Can you work these out from the model? Positions are in its coordinate system, mm. A direction names the side the tool comes from. Give positions to 0.01 mm unless a question says otherwise; leave off trailing zeros. Order: outer loops, then holes, each group sorted by start corner. A loop starts at its lowest first (then second) coordinate and runs counter-clockwise, first axis right, second up.
Item 1: I'm going to push flat-ended pins straight in: pin 1 Ø1.2 at (x, z) = (-32.5, 8.5) entering from +Y; pin 2 Ø8 at (y, z) = (-13, 0.5) entering from -X; pin 3 Ø5.5 at (y, z) = (30.5, 8.5) entering from -X. Where does each tip first touch, or does it pass through?
Item 2: Which directions (+Z, -Z, +X, -X, +Y, -Y) give clear straight access to the entire face, cutting with the end or side of a thin tool? Please do faces 4 (the flat face through (-21, -55, 14.5)), 5 (the flat face through (-21, -73, 16)), 6 (the flat face through (-33, -36.914, 10)), 7 (the flat face through (-21, 7, 4)).
Item 3: I want a section at A-A, the plane y = 16.5. Write out the boundary of the cut face in (x, z), then the cut area to 3 significant figures.
Item 4: If we mould it in two halves opening along X, with no side actions, what happens to faces 1 (the flat face through (0, 48.37, 11)), 2 (the flat face through (22.5, -15, 16)), 3 (the cylindrical face through (-16.291, -75.643, 9.93))? For each: +X half, -X half, draft (parallel to the pull), parting line (faces both ways), or undercut.
Item 5: If I drill on line 1 along X through (y, z) = (-12, -2.75); line 2 along X through (y, z) = (0, 12.25); line 3 along Y through (x, z) = (14.5, 1.95), over which ranges is the centre line in solid material (lowest first)?
```python
from build123d import *

# Parameters (mm, degrees)
CROQUIS1_W               = 38
CROQUIS1_H               = 81
CROQUIS1_W_2             = 27
CROQUIS1_H_2             = 72
CROQUIS1_H_3             = 38
CROQUIS1_R               = 3.5
SALIENTE_EXTRUIR1_DEPTH  = 5
CROQUIS2_W               = 38
CROQUIS2_H               = 81
CROQUIS2_W_2             = 27
CROQUIS2_H_2             = 72
SALIENTE_EXTRUIR2_DEPTH  = 5
SALIENTE_EXTRUIR9_START  = -1
SALIENTE_EXTRUIR9_DEPTH  = 1
SALIENTE_EXTRUIR10_DEPTH = 11
SALIENTE_EXTRUIR11_DEPTH = 10
REDONDEO1_R              = 1
REDONDEO2_R              = 1
REDONDEO3_R              = 1
CROQUIS6_W               = 6
CROQUIS6_H               = 9
CORTAR_EXTRUIR1_DEPTH    = 8
CROQUIS7_W               = 6
CROQUIS7_H               = 9
CROQUIS7_R               = 2.5
SALIENTE_EXTRUIR12_DEPTH = 3
SALIENTE_EXTRUIR13_DEPTH = 11
REDONDEO4_R              = 5
CROQUIS9_R               = 0.6
CORTAR_EXTRUIR2_DEPTH    = 80
SALIENTE_EXTRUIR14_START = -2.5
CROQUIS10_R              = 0.6
SALIENTE_EXTRUIR14_DEPTH = 2.5
CROQUIS11_R              = 4
CROQUIS11_R_2            = 3.5
CROQUIS11_R_3            = 2.5
CROQUIS11_R_4            = 2
CORTAR_EXTRUIR3_DEPTH    = 1
SALIENTE_EXTRUIR15_DEPTH = 3
CROQUIS14_R              = 1.5
CORTAR_EXTRUIR4_DEPTH    = 14
CROQUIS16_W              = 3.5
CROQUIS16_H              = 3
SALIENTE_EXTRUIR16_DEPTH = 4
CROQUIS25_R              = 3
CROQUIS25_R_2            = 1.5
SALIENTE_EXTRUIR21_DEPTH = 18
CROQUIS26_R              = 1.5
CORTAR_EXTRUIR7_DEPTH    = 18
CROQUIS28_R              = 1
CORTAR_EXTRUIR8_DEPTH    = 4


with BuildPart() as part:
    # Croquis1 → Saliente-Extruir1 (new body)
    # profile 1 of 5: a face of its own
    with BuildSketch(Plane.XY):
        Rectangle(CROQUIS1_W, CROQUIS1_H)
        Rectangle(CROQUIS1_W_2, CROQUIS1_H_2, mode=Mode.SUBTRACT)
    # profile 2 of 5: a face of its own
    with BuildSketch(Plane.XY):
        with Locations((0, -59.5)):
            Rectangle(CROQUIS1_W, CROQUIS1_H_3)
        with Locations((-9.5, -69)):
            Circle(CROQUIS1_R, mode=Mode.SUBTRACT)
        with Locations((9.5, -59.5)):
            Circle(CROQUIS1_R, mode=Mode.SUBTRACT)
        with Locations((-9.5, -50)):
            Circle(CROQUIS1_R, mode=Mode.SUBTRACT)
    # profile 3 of 5: a face of its own
    with BuildSketch(Plane.XY):
        with BuildLine():
            ThreePointArc((19, -78.5), (26.870057685, -59.5), (19, -40.5))
            Line((19, -40.5), (19, -78.5))
        make_face()
    # profile 4 of 5: a face of its own
    with BuildSketch(Plane.XY):
        with BuildLine():
            Line((19, -78.5), (-19, -78.5))
            ThreePointArc((-19, -78.5), (0, -86.370057685), (19, -78.5))
        make_face()
    # profile 5 of 5: a face of its own
    with BuildSketch(Plane.XY):
        with BuildLine():
            Line((-19, -78.5), (-19, -40.5))
            ThreePointArc((-19, -40.5), (-26.870057685, -59.5), (-19, -78.5))
        make_face()
    extrude(amount=SALIENTE_EXTRUIR1_DEPTH)

    # Croquis2 → Saliente-Extruir2 (add)
    with BuildSketch(Plane(origin=(0, 0, 0), x_dir=(-1, 0, 0), z_dir=(0, 0, -1))):
        Rectangle(CROQUIS2_W, CROQUIS2_H)
        Rectangle(CROQUIS2_W_2, CROQUIS2_H_2, mode=Mode.SUBTRACT)
    extrude(amount=SALIENTE_EXTRUIR2_DEPTH)

    # Croquis3 → Saliente-Extruir9 (add)
    with BuildSketch(Plane.XY.offset(5).offset(SALIENTE_EXTRUIR9_START)):
        with BuildLine():
            Line((26.870057685, -59.5), (26.870057685, 40.5))
            Line((26.870057685, 40.5), (19, 48.370057685))
            Line((19, 48.370057685), (-19, 48.370057685))
            Line((-19, 48.370057685), (-26.870057685, 40.5))
            Line((-26.870057685, 40.5), (-26.870057685, -59.5))
            ThreePointArc((-26.870057685, -59.5), (0, -86.370057685), (26.870057685, -59.5))
        make_face()
        with BuildLine():
            Line((19, -59.5), (19, 40.5))
            Line((19, 40.5), (-19, 40.5))
            Line((-19, 40.5), (-19, -59.5))
            ThreePointArc((-19, -59.5), (0, -78.5), (19, -59.5))
        make_face(mode=Mode.SUBTRACT)
    extrude(amount=SALIENTE_EXTRUIR9_DEPTH)

    # Croquis4 → Saliente-Extruir10 (add)
    with BuildSketch(Plane(origin=(0, 0, 4), x_dir=(-1, 0, 0), z_dir=(0, 0, -1))):
        with BuildLine():
            Line((19, 40.5), (19, -40.5))
            ThreePointArc((19, -40.5), (24.824696333, -49.217274097), (26.870057685, -59.5))
            Line((26.870057685, -59.5), (26.870057685, 40.5))
            Line((26.870057685, 40.5), (19, 48.370057685))
            Line((19, 48.370057685), (-19, 48.370057685))
            Line((-19, 48.370057685), (-26.870057685, 40.5))
            Line((-26.870057685, 40.5), (-26.870057685, -59.5))
            ThreePointArc((-26.870057685, -59.5), (-24.824696333, -49.217274097), (-19, -40.5))
            Line((-19, -40.5), (-19, 40.5))
            Line((-19, 40.5), (19, 40.5))
        make_face()
    extrude(amount=-SALIENTE_EXTRUIR10_DEPTH)

    # Croquis5 → Saliente-Extruir11 (add)
    with BuildSketch(Plane.XY.offset(5)):
        with BuildLine():
            Line((-19, -59.5), (-19, -69))
            ThreePointArc((-19, -69), (-16.217514421, -75.717514421), (-9.5, -78.5))
            Line((-9.5, -78.5), (9.5, -78.5))
            ThreePointArc((9.5, -78.5), (16.217514421, -75.717514421), (19, -69))
            Line((19, -69), (19, -59.5))
            Line((19, -59.5), (19, -40.5))
            ThreePointArc((19, -40.5), (0, -86.370057685), (-19, -40.5))
            Line((-19, -40.5), (-19, -59.5))
        make_face()
    extrude(amount=SALIENTE_EXTRUIR11_DEPTH)

    # Redondeo1
    redondeo1_edges = [part.edges().sort_by_distance(p)[0] for p in [
        (19, -40.5, -2.5),
        (-19, -40.5, -2.5),
        (19, 40.5, -0.5),
        (-19, 40.5, -0.5),
    ]]
    fillet(redondeo1_edges, radius=REDONDEO1_R)

    # Redondeo2
    redondeo2_edges = [part.edges().sort_by_distance(p)[0] for p in [
        (-19, -0.5, 4),
        (0, 40.5, 4),
        (-18.707106781, 40.207106781, 4),
        (18.707106781, 40.207106781, 4),
        (19, -0.5, 4),
    ]]
    fillet(redondeo2_edges, radius=REDONDEO2_R)

    # Redondeo3
    redondeo3_edges = [part.edges().sort_by_distance(p)[0] for p in [
        (19, 48.370057685, 9.5),
        (26.870057685, 40.5, 9.5),
        (-26.870057685, 40.5, 9.5),
        (-19, 48.370057685, 9.5),
    ]]
    fillet(redondeo3_edges, radius=REDONDEO3_R)

    # Croquis6 → Cortar-Extruir1 (cut)
    with BuildSketch(Plane.ZY.offset(26.870057685)):
        with Locations((11.5, -55)):
            Rectangle(CROQUIS6_W, CROQUIS6_H)
    extrude(amount=-CORTAR_EXTRUIR1_DEPTH, mode=Mode.SUBTRACT)

    # Croquis7 → Saliente-Extruir12 (add)
    with BuildSketch(Plane.ZY.offset(26.870057685)):
        with Locations((11.5, -55)):
            Rectangle(CROQUIS7_W, CROQUIS7_H)
        with Locations((11.5, -55)):
            Circle(CROQUIS7_R, mode=Mode.SUBTRACT)
    extrude(amount=-SALIENTE_EXTRUIR12_DEPTH)

    # Croquis8 → Saliente-Extruir13 (add)
    with BuildSketch(Plane.ZY.offset(26.870057685)):
        Polygon((15, 40.085786438), (4, 40.085786438), (4, 37.085786438), (9.5, 37.085786438), (15, 37.085786438), align=None)
        Polygon((9.5, 15.085786438), (4, 15.085786438), (4, 12.085786438), (9.5, 12.085786438), (15, 12.085786438), (15, 15.085786438), align=None)
        Polygon((9.5, -10.914213562), (4, -10.914213562), (4, -13.914213562), (9.5, -13.914213562), (15, -13.914213562), (15, -10.914213562), align=None)
        Polygon((9.5, -36.914213562), (4, -36.914213562), (4, -39.914213562), (15, -39.914213562), (15, -36.914213562), align=None)
    extrude(amount=SALIENTE_EXTRUIR13_DEPTH)

    # Redondeo4
    redondeo4_edges = [part.edges().sort_by_distance(p)[0] for p in [
        (-37.870057685, 38.585786438, 4),
        (-37.870057685, 38.585786438, 15),
        (-37.870057685, 13.585786438, 4),
        (-37.870057685, 13.585786438, 15),
        (-37.870057685, -12.414213562, 4),
        (-37.870057685, -12.414213562, 15),
        (-37.870057685, -38.414213562, 4),
        (-37.870057685, -38.414213562, 15),
    ]]
    fillet(redondeo4_edges, radius=REDONDEO4_R)

    # Croquis9 → Cortar-Extruir2 (cut)
    with BuildSketch(Plane(origin=(0, 40.085786438, 0), x_dir=(1, 0, 0), z_dir=(0, 1, 0))):
        with Locations(Location((-32.370057685, -9.5, 0), (0, 0, 270))):
            Circle(CROQUIS9_R)
    extrude(amount=-CORTAR_EXTRUIR2_DEPTH, mode=Mode.SUBTRACT)

    # Croquis10 → Saliente-Extruir14 (add)
    with BuildSketch(Plane.XZ.offset(39.914213562).offset(SALIENTE_EXTRUIR14_START)):
        with Locations(Location((-32.370057685, 9.5, 0), (0, 0, 90))):
            Circle(CROQUIS10_R)
    extrude(amount=SALIENTE_EXTRUIR14_DEPTH)

    # Croquis11 → Cortar-Extruir3 (cut)
    # profile 1 of 2: a face of its own
    with BuildSketch(Plane(origin=(0, -36.914213562, 0), x_dir=(1, 0, 0), z_dir=(0, 1, 0))):
        with Locations(Location((-32.370057685, -9.5, 0), (0, 0, 270))):
            Circle(CROQUIS11_R)
        with Locations(Location((-32.370057685, -9.5, 0), (0, 0, 270))):
            Circle(CROQUIS11_R_2, mode=Mode.SUBTRACT)
    # profile 2 of 2: a face of its own
    with BuildSketch(Plane(origin=(0, -36.914213562, 0), x_dir=(1, 0, 0), z_dir=(0, 1, 0))):
        with Locations(Location((-32.370057685, -9.5, 0), (0, 0, 270))):
            Circle(CROQUIS11_R_3)
        with Locations(Location((-32.370057685, -9.5, 0), (0, 0, 270))):
            Circle(CROQUIS11_R_4, mode=Mode.SUBTRACT)
    extrude(amount=-CORTAR_EXTRUIR3_DEPTH, mode=Mode.SUBTRACT)

    # Croquis13 → Saliente-Extruir15 (add)
    with BuildSketch(Plane.XY.offset(15)):
        Polygon((-19, -65.5), (-19, 40.5), (-22.5, 40.5), (-22.5, -69), (-19, -69), align=None)
        Polygon((22.5, 40.5), (19, 40.5), (19, -65.5), (19, -69), (22.5, -69), align=None)
        with BuildLine():
            Line((-19, 40.5), (19, 40.5))
            Line((19, 40.5), (22.5, 40.5))
            Line((22.5, 40.5), (22.5, 44.870057685))
            Line((22.5, 44.870057685), (19.292893219, 48.077164466))
            ThreePointArc((19.292893219, 48.077164466), (18.96846987, 48.293937218), (18.585786438, 48.370057685))
            Line((18.585786438, 48.370057685), (-18.585786438, 48.370057685))
            ThreePointArc((-18.585786438, 48.370057685), (-18.96846987, 48.293937218), (-19.292893219, 48.077164466))
            Line((-19.292893219, 48.077164466), (-22.5, 44.870057685))
            Line((-22.5, 44.870057685), (-22.5, 40.5))
            Line((-22.5, 40.5), (-19, 40.5))
        make_face()
    extrude(amount=SALIENTE_EXTRUIR15_DEPTH)

    # Croquis14 → Cortar-Extruir4 (cut)
    with BuildSketch(Plane(origin=(0, 0, 4), x_dir=(-1, 0, 0), z_dir=(0, 0, -1))):
        with Locations((10, 45.370057685)):
            Circle(CROQUIS14_R)
        with Locations(Location((-10, 45.370057685, 0), (0, 0, 180))):
            Circle(CROQUIS14_R)
    extrude(amount=-CORTAR_EXTRUIR4_DEPTH, mode=Mode.SUBTRACT)

    # Croquis16 → Saliente-Extruir16 (add)
    with BuildSketch(Plane(origin=(0, -69, 0), x_dir=(-1, 0, 0), z_dir=(0, -1, 0))):
        with Locations((20.75, -16.5)):
            Rectangle(CROQUIS16_W, CROQUIS16_H)
        with Locations((-20.75, -16.5)):
            Rectangle(CROQUIS16_W, CROQUIS16_H)
    extrude(amount=SALIENTE_EXTRUIR16_DEPTH)

    # Croquis25 → Saliente-Extruir21 (add)
    with BuildSketch(Plane.XY.offset(18)):
        with Locations((0, -70.629942315)):
            Circle(CROQUIS25_R)
        with Locations((0, -70.629942315)):
            Circle(CROQUIS25_R_2, mode=Mode.SUBTRACT)
    extrude(amount=-SALIENTE_EXTRUIR21_DEPTH)

    # Croquis26 → Cortar-Extruir7 (cut)
    with BuildSketch(Plane.XY.offset(18)):
        with Locations((0, -70.629942315)):
            Circle(CROQUIS26_R)
    extrude(amount=-CORTAR_EXTRUIR7_DEPTH, mode=Mode.SUBTRACT)

    # Croquis28 → Cortar-Extruir8 (cut)
    with BuildSketch(Plane.XY.offset(5)):
        with Locations((-16.5, 38)):
            Circle(CROQUIS28_R)
        with Locations((14.5, 38)):
            Circle(CROQUIS28_R)
        with Locations((14.5, -37)):
            Circle(CROQUIS28_R)
        with Locations((-16.5, -37)):
            Circle(CROQUIS28_R)
    extrude(amount=-CORTAR_EXTRUIR8_DEPTH, mode=Mode.SUBTRACT)


solid = part.part
```
Results list:
1. pin 1: stops at y = 40.09
1. pin 2: stops at x = -35.05
1. pin 3: stops at x = -26.87
2. face 4: none
2. face 5: +Z, -X, -Y
2. face 6: +Z, -Z, -X
2. face 7: -Z, +Y
3. outline: (-26.87, 4) - (-20, 4) arc R1 cw to (-19, 3) - (-19, -5) - (-13.5, -5) - (-13.5, 5) - (-19, 5) - (-19, 18) - (-22.5, 18) - (-22.5, 15) - (-26.87, 15) - close; (13.5, -5) - (19, -5) - (19, 3) arc R1 cw to (20, 4) - (26.87, 4) - (26.87, 15) - (22.5, 15) - (22.5, 18) - (19, 18) - (19, 5) - (13.5, 5) - close
3. area: 305 mm2
4. face 1: draft
4. face 2: +X half
4. face 3: undercut
5. line 1: x = -19 to -13.5, 13.5 to 19
5. line 2: x = -26.87 to -19, 19 to 26.87
5. line 3: y = -82.12 to -38, -36 to 37, 39 to 40.5
